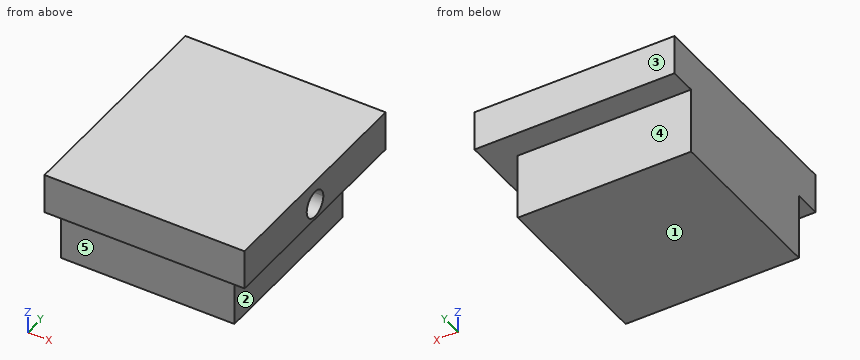
```python
from build123d import *

# Parameters (mm, degrees)
F0_W     = 13
F0_H     = 13
F1_DEPTH = 8
F3_DEPTH = 3
F5_DEPTH = 10


with BuildPart() as f1:
    # F0 (on Top) → F1 (new body)
    with BuildSketch(Plane.XY):
        with Locations((6.5, 6.5)):
            Rectangle(F0_W, F0_H)
    extrude(amount=F1_DEPTH)

    # F2 (on face) → F3 (join)
    with BuildSketch(Plane.XY.offset(8)):
        Polygon((13, 0), (0, 0), (0, -2), (15, -2), (15, 15), (0, 15), (0, 13), (13, 13), align=None)
    extrude(amount=-F3_DEPTH)

    # F4 (on face) → F5 (cut)
    with BuildSketch(Plane.YZ.offset(15)):
        with BuildLine():
            ThreePointArc((7.5, 6.2), (7.207107, 6.907107), (6.5, 7.2))
            ThreePointArc((6.5, 7.2), (5.792893, 5.492893), (7.5, 6.2))
        make_face()
    extrude(amount=-F5_DEPTH, mode=Mode.SUBTRACT)


solid = f1.part
```
The listing builds one solid part. Answer for the finished solid, in the listing's coordinates (mm). Face numbers are marked on the shaded views. A direction names the side the tool comes from. Coordinates: 2 decimals unless noted, no trailing zeros. Write each loop counter-clockwise with the first axis right and the second up, starting at its lowest first coordinate (ties: lowest second). Pieces come first, ordered by that corner, then holes. Notation, with made-up numbers: (39, 67.5) - (47, 67.5) arc R31 ccw to (47, 93.5) - close; hole circle Ø10 at (59, 78). An arc over 180 degrees is marked (long way). Return JSON: item names as keys, results as strings. Group by question number.
Q1. Find the intervals of material crossed by line 1 along Y through (x, z) = (11.25, 6.2); line 2 along Z through (x, y) = (12, 6.5); line 3 along X through (y, z) = (0.5, 0.5), in increasing order. Write a range as [from, to].
Q2. The part is cut by section D-D on z = 3.75. Write down the section's boundary in (x, y), and give its area (3 significant figures).
Q3. The part is cut by section B-B on x = 1.5. Write down the section's boundary in (y, z), and give its area (3 significant figures).
Q4. Flat-ended cylindrical pins translate along their axes: pin 1 Ø0.6 at (y, z) = (6.5, 6) entering from +X; pin 2 Ø1.5 at (x, z) = (7.5, 1.5) entering from +Y; pin 3 Ø2.5 at (y, z) = (3.5, 3.5) entering from +X. Find the tip coordinate at first contact, or state that the pin passes through.
Q5. The part is cut by section A-A on x = 11.5. Write down the section's boundary in (y, z).
Q6. Which of the six approach directions +Z, -Z, +X, -X, +Y, -Y give full straight-line access (tool end or side, diameter ignored) to the marked faces 1, 2, 3, 4 and 5?
Q7. The part is cut by section C-C on y = 6.25. Write down the section's boundary in (x, z).
Evaluation:
{
 "1": {"line 1": "y = [-2, 5.5], [7.5, 15]", "line 2": "z = [0, 5.2], [7.2, 8]", "line 3": "x = [0, 13]"},
 "2": {"outline": "(0, 0) - (13, 0) - (13, 13) - (0, 13) - close", "area": "169 mm2"},
 "3": {"outline": "(-2, 5) - (0, 5) - (0, 0) - (13, 0) - (13, 5) - (15, 5) - (15, 8) - (-2, 8) - close", "area": "116 mm2"},
 "4": {"pin 1": "stops at x = 5", "pin 2": "stops at y = 13", "pin 3": "stops at x = 13"},
 "5": {"outline": "(-2, 5) - (0, 5) - (0, 0) - (13, 0) - (13, 5) - (15, 5) - (15, 8) - (-2, 8) - close; hole circle Ø2 at (6.5, 6.2)"},
 "6": {"face 1": "-Z, +X, -X, +Y, -Y", "face 2": "-Z, +X, +Y, -Y", "face 3": "+Z, -Z, +X, -X, +Y", "face 4": "-Z, +X, -X, +Y", "face 5": "-Z, +X, -X, -Y"},
 "7": {"outline": "(0, 0) - (13, 0) - (13, 5) - (15, 5) - (15, 5.23) - (5, 5.23) - (5, 7.17) - (15, 7.17) - (15, 8) - (0, 8) - close"}
}
